from build123d import *

# Parameters (mm, degrees)
F1_DEPTH = 5


with BuildPart() as f1:
    # F0 (on Top) → F1 (new body)
    with BuildSketch(Plane.XY):
        with BuildLine():
            Line((0, 12.222), (0, 1.778))
            ThreePointArc((0, 1.778), (0.520764, 0.520764), (1.778, 0))
            Line((1.778, 0), (12.222, 0))
            ThreePointArc((12.222, 0), (13.479236, 0.520764), (14, 1.778))
            Line((14, 1.778), (14, 12.222))
            ThreePointArc((14, 12.222), (13.479236, 13.479236), (12.222, 14))
            Line((12.222, 14), (10.1, 14))
            Line((10.1, 14), (10.1, 4))
            Line((10.1, 4), (3.9, 4))
            Line((3.9, 4), (3.9, 14))
            Line((3.9, 14), (1.778, 14))
            ThreePointArc((1.778, 14), (0.520764, 13.479236), (0, 12.222))
        make_face()
    extrude(amount=F1_DEPTH)


solid = f1.part
Geometry: final body of the model. Coordinates: model frame, mm. A direction names the side the tool comes from. Round coordinates to 2 decimals unless told otherwise and drop trailing zeros. Loops run counter-clockwise (first coordinate to the right, second up) from the corner with the lowest first, then second, coordinate; pieces in that order, holes last. Notation, with made-up numbers: (-33.75, -0.75) - (-11.75, -0.75) arc R14 cw to (-11.75, 4.25) - close; hole circle Ø3 at (39, 2). An arc over 180 degrees is marked (long way). Write each question's results on one line, items separated by ' | '. Start each with the question number.
1) Cut plane B-B on z = 1.35. Return loops of the section in (x, y).
2) Cut plane D-D on y = 1. Return loops of the section in (x, z).
3) Mould query, pull axis X, two halves, no side actions, for faces 1 (the face through (3.9, 9, 2)), 2 (the face through (7, 0, 2)), 3 (the face through (7, 4, 2)), 4 (the face through (14, 7, 2)). Classes: released by +X, released by -X, zero draft, split by the parting line, or undercut.
4) Cut plane A-A on y = 7. Return loops of the section in (x, z), then the cut area to 3 significant figures.
5) Access query for faces 5 (the face through (10.1, 9, 2)), 6 (the face through (13.49, 13.47, 2.46)). Directions: +Z, -Z, +X, -X, +Y, -Y. A direction counts if a zero-diameter tool reaches every point of the face in a straight line with its end or side. Return the directions, or none.
6) Line query: probe 1 along X at (y, z) = (6.25, 2.7); probe 2 along Y at (x, z) = (5, 3.95); probe 3 along Y at (x, z) = (12.75, 1.85). Output: solid intervals per line, ascending. Write a range as [from, to].
7) First-contact query: P1, Ø1, axis at x = 6, y = 10.5, coming from the -Z side; P2, Ø3, axis at x = 8.5, z = 2, coming from the +Y side. Flat tips, straight axial feed; report the tip coordinate or a pass-through.
8) Cut plane C-C on x = 5.5. Return loops of the section in (y, z), then the cut area to 3 significant figures.
Verdict:
1) outline: (0, 1.78) arc R1.78 ccw to (1.78, 0) - (12.22, 0) arc R1.78 ccw to (14, 1.78) - (14, 12.22) arc R1.78 ccw to (12.22, 14) - (10.1, 14) - (10.1, 4) - (3.9, 4) - (3.9, 14) - (1.78, 14) arc R1.78 ccw to (0, 12.22) - close
2) outline: (0.18, 0) - (13.82, 0) - (13.82, 5) - (0.18, 5) - close
3) face 1: undercut | face 2: zero draft | face 3: undercut | face 4: released by +X
4) outline: (0, 0) - (3.9, 0) - (3.9, 5) - (0, 5) - close; (10.1, 0) - (14, 0) - (14, 5) - (10.1, 5) - close | area: 39.0 mm2
5) face 5: +Z, -Z, +Y | face 6: +Z, -Z, +X, +Y
6) probe 1: x = [0, 3.9], [10.1, 14] | probe 2: y = [0, 4] | probe 3: y = [0.08, 13.92]
7) P1: passes through | P2: stops at y = 4
8) outline: (0, 0) - (4, 0) - (4, 5) - (0, 5) - close | area: 20.0 mm2
